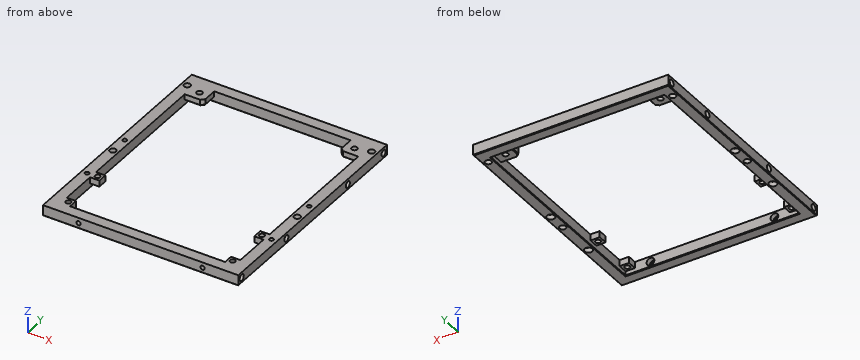
```python
from build123d import *

# Parameters (mm, degrees)
SKETCH1_W                       = 126
SKETCH1_H                       = 150
SKETCH1_W_2                     = 112
SKETCH1_H_2                     = 136
BOSS_EXTRUDE1_DEPTH             = 7
SKETCH2_R                       = 2.05
CUT_EXTRUDE1_DEPTH              = 6
SKETCH3_R                       = 1.35
CUT_EXTRUDE2_DEPTH              = 8
SKETCH4_R                       = 2.5
CUT_EXTRUDE3_DEPTH              = 3
SKETCH5_R                       = 1.35
CUT_EXTRUDE4_DEPTH              = 8
SKETCH6_R                       = 2.5
CUT_EXTRUDE5_DEPTH              = 3
SKETCH7_R                       = 2.05
CUT_EXTRUDE6_DEPTH              = 8
CUT_EXTRUDE7_DEPTH              = 0.2
SKETCH9_W                       = 2.7
SKETCH9_H                       = 2.7
CUT_EXTRUDE8_DEPTH              = 0.2
SKETCH10_W                      = 6
SKETCH10_H                      = 6
BOSS_EXTRUDE2_DEPTH             = 4
SKETCH11_R                      = 1.65
CUT_EXTRUDE9_DEPTH              = 5
CHAMFER1_SIZE                   = 0.4
CHAMFER2_SIZE                   = 0.4
SKIZZE2_W                       = 12
SKIZZE2_H                       = 11
SKIZZE2_R                       = 1.8
AUFSATZ_LINEAR_AUSTRAGEN1_DEPTH = 4
FASE1_SIZE                      = 2
FASE2_SIZE                      = 0.5


with BuildPart() as part:
    # Sketch1 → Boss-Extrude1 (new body)
    with BuildSketch(Plane.XY):
        Rectangle(SKETCH1_W, SKETCH1_H)
        Rectangle(SKETCH1_W_2, SKETCH1_H_2, mode=Mode.SUBTRACT)
    extrude(amount=BOSS_EXTRUDE1_DEPTH)

    # Sketch2 → Cut-Extrude1 (cut)
    with BuildSketch(Plane.ZY.offset(63)):
        with Locations((3.5, -71.5)):
            Circle(SKETCH2_R)
        with Locations((3.5, 71.5)):
            Circle(SKETCH2_R)
        with Locations((3.5, 35.5)):
            Circle(SKETCH2_R)
        with Locations((3.5, -26.5)):
            Circle(SKETCH2_R)
    cut_extrude1 = extrude(amount=-CUT_EXTRUDE1_DEPTH, mode=Mode.SUBTRACT)

    # Mirror1: Cut-Extrude1 across plane
    add(cut_extrude1.mirror(Plane(origin=(0, 0, 0), x_dir=(0, 0, 1), z_dir=(1, 0, 0))), mode=Mode.SUBTRACT)

    # Sketch3 → Cut-Extrude2 (cut, through all)
    with BuildSketch(Plane(origin=(0, -68, 0), x_dir=(1, 0, 0), z_dir=(0, 1, 0))):
        with Locations((40, -3.5)):
            Circle(SKETCH3_R)
        with Locations((-40, -3.5)):
            Circle(SKETCH3_R)
    extrude(amount=-CUT_EXTRUDE2_DEPTH, mode=Mode.SUBTRACT)

    # Sketch4 → Cut-Extrude3 (cut)
    with BuildSketch(Plane(origin=(0, -68, 0), x_dir=(1, 0, 0), z_dir=(0, 1, 0))):
        with Locations((40, -3.5)):
            Circle(SKETCH4_R)
        with Locations((-40, -3.5)):
            Circle(SKETCH4_R)
    extrude(amount=-CUT_EXTRUDE3_DEPTH, mode=Mode.SUBTRACT)

    # Sketch5 → Cut-Extrude4 (cut, through all)
    with BuildSketch(Plane(origin=(0, 0, 0), x_dir=(-1, 0, 0), z_dir=(0, 0, -1))):
        with Locations((-59.5, 2)):
            Circle(SKETCH5_R)
        with Locations((59.5, 2)):
            Circle(SKETCH5_R)
        with Locations((-59.5, -36)):
            Circle(SKETCH5_R)
        with Locations((59.5, -36)):
            Circle(SKETCH5_R)
    extrude(amount=-CUT_EXTRUDE4_DEPTH, mode=Mode.SUBTRACT)

    # Sketch6 → Cut-Extrude5 (cut)
    with BuildSketch(Plane(origin=(0, 0, 0), x_dir=(-1, 0, 0), z_dir=(0, 0, -1))):
        with Locations((-59.5, 2)):
            Circle(SKETCH6_R)
        with Locations((59.5, 2)):
            Circle(SKETCH6_R)
        with Locations((-59.5, -36)):
            Circle(SKETCH6_R)
        with Locations((59.5, -36)):
            Circle(SKETCH6_R)
    extrude(amount=-CUT_EXTRUDE5_DEPTH, mode=Mode.SUBTRACT)

    # Sketch7 → Cut-Extrude6 (cut, through all)
    with BuildSketch(Plane(origin=(0, 0, 0), x_dir=(-1, 0, 0), z_dir=(0, 0, -1))):
        with Locations((-59.5, 65)):
            Circle(SKETCH7_R)
        with Locations((-59.5, -10)):
            Circle(SKETCH7_R)
    cut_extrude6 = extrude(amount=-CUT_EXTRUDE6_DEPTH, mode=Mode.SUBTRACT)

    # Mirror2: Cut-Extrude6 across plane
    add(cut_extrude6.mirror(Plane(origin=(0, 0, 0), x_dir=(0, 0, 1), z_dir=(1, 0, 0))), mode=Mode.SUBTRACT)

    # Sketch8 → Cut-Extrude7 (cut)
    with BuildSketch(Plane(origin=(0, 0, 3), x_dir=(-1, 0, 0), z_dir=(0, 0, -1))):
        with BuildLine():
            Line((-60.85, -0.104162541), (-60.85, 4.104162541))
            ThreePointArc((-60.85, 4.104162541), (-59.5, 4.5), (-58.15, 4.104162541))
            Line((-58.15, 4.104162541), (-58.15, -0.104162541))
            ThreePointArc((-58.15, -0.104162541), (-59.5, -0.5), (-60.85, -0.104162541))
        make_face()
        with BuildLine():
            Line((-60.85, -38.104162541), (-60.85, -33.895837459))
            ThreePointArc((-60.85, -33.895837459), (-59.5, -33.5), (-58.15, -33.895837459))
            Line((-58.15, -33.895837459), (-58.15, -38.104162541))
            ThreePointArc((-58.15, -38.104162541), (-59.5, -38.5), (-60.85, -38.104162541))
        make_face()
    cut_extrude7 = extrude(amount=-CUT_EXTRUDE7_DEPTH, mode=Mode.SUBTRACT)

    # Sketch9 → Cut-Extrude8 (cut)
    with BuildSketch(Plane(origin=(0, 0, 3.2), x_dir=(-1, 0, 0), z_dir=(0, 0, -1))):
        with Locations((-59.5, 2)):
            Rectangle(SKETCH9_W, SKETCH9_H)
        with Locations((-59.5, -36)):
            Rectangle(SKETCH9_W, SKETCH9_H)
    cut_extrude8 = extrude(amount=-CUT_EXTRUDE8_DEPTH, mode=Mode.SUBTRACT)

    # Mirror3: Cut-Extrude7, Cut-Extrude8 across plane
    add(cut_extrude7.mirror(Plane(origin=(0, 0, 0), x_dir=(0, 0, 1), z_dir=(1, 0, 0))), mode=Mode.SUBTRACT)
    add(cut_extrude8.mirror(Plane(origin=(0, 0, 0), x_dir=(0, 0, 1), z_dir=(1, 0, 0))), mode=Mode.SUBTRACT)

    # Sketch10 → Boss-Extrude2 (add)
    with BuildSketch(Plane.XY.offset(7)):
        with Locations((53, -65)):
            Rectangle(SKETCH10_W, SKETCH10_H)
        with Locations((53, -35.5)):
            Rectangle(SKETCH10_W, SKETCH10_H)
    boss_extrude2 = extrude(amount=-BOSS_EXTRUDE2_DEPTH)

    # Sketch11 → Cut-Extrude9 (cut, through all)
    with BuildSketch(Plane(origin=(0, 0, 3), x_dir=(-1, 0, 0), z_dir=(0, 0, -1))):
        with Locations((-53, -35.5)):
            Circle(SKETCH11_R)
        with Locations((-53, -65)):
            Circle(SKETCH11_R)
    cut_extrude9 = extrude(amount=-CUT_EXTRUDE9_DEPTH, mode=Mode.SUBTRACT)

    # Mirror4: Boss-Extrude2, Cut-Extrude9 across plane
    add(boss_extrude2.mirror(Plane(origin=(0, 0, 0), x_dir=(0, 0, 1), z_dir=(1, 0, 0))))
    add(cut_extrude9.mirror(Plane(origin=(0, 0, 0), x_dir=(0, 0, 1), z_dir=(1, 0, 0))), mode=Mode.SUBTRACT)

    # Chamfer1
    chamfer1_edges = [part.edges().sort_by_distance(p)[0] for p in [
        (56, 0, 0),
        (0, 68, 0),
        (-56, 0, 0),
        (0, -68, 0),
    ]]
    chamfer(chamfer1_edges, length=CHAMFER1_SIZE)

    # Chamfer2
    chamfer2_edges = [part.edges().sort_by_distance(p)[0] for p in [
        (0, -75, 0),
        (-63, 0, 0),
        (0, 75, 0),
        (63, 0, 0),
    ]]
    chamfer(chamfer2_edges, length=CHAMFER2_SIZE)

    # Skizze2 → Aufsatz-Linear austragen1 (add)
    with BuildSketch(Plane.XY.offset(7)):
        with Locations((-50, 62.5)):
            Rectangle(SKIZZE2_W, SKIZZE2_H)
        with Locations((-50, 62.5)):
            Circle(SKIZZE2_R, mode=Mode.SUBTRACT)
        with Locations((50, 62.5)):
            Rectangle(SKIZZE2_W, SKIZZE2_H)
        with Locations((50, 62.5)):
            Circle(SKIZZE2_R, mode=Mode.SUBTRACT)
    extrude(amount=-AUFSATZ_LINEAR_AUSTRAGEN1_DEPTH)

    # Fase1
    fase1_edges = [part.edges().sort_by_distance(p)[0] for p in [
        (-44, 57, 5),
        (44, 57, 5),
    ]]
    chamfer(fase1_edges, length=FASE1_SIZE)

    # Fase2
    fase2_edges = [part.edges().sort_by_distance(p)[0] for p in [
        (-51, 57, 3),
        (44, 63.5, 3),
        (-44, 63.5, 3),
        (-45, 58, 3),
        (51, 57, 3),
        (45, 58, 3),
    ]]
    chamfer(fase2_edges, length=FASE2_SIZE)


solid = part.part
```
Check sheet for the modelled part. Datum: model origin and axes. Units: mm. Round coordinates to 2 decimals unless told otherwise and drop trailing zeros. Write each loop counter-clockwise with the first axis right and the second up, starting at its lowest first coordinate (ties: lowest second). Pieces come first, ordered by that corner, then holes. Notation, with made-up numbers: (77, 64) -> (133, 64) arc R27 cw to (133, 96) -> close; hole circle Ø10 at (58, 19). An arc over 180 degrees is marked (long way). Put each result on its own line as item: value.
(1) Material ranges on line 1 (X direction, y = 2, z = 0.95); line 2 (Y direction, x = -22.5, z = 6); line 3 (X direction, y = 60.5, z = 1), recorded low to high.
Values found:
line 1: x = -63 to -62, -57 to -56, 56 to 57, 62 to 63
line 2: y = -75 to -68, 68 to 75
line 3: x = -63 to -56, 56 to 63
(2) Go/stop test with flat-tipped pins: pin 1 Ø1.1 at (x, y) = (-60.5, -36.5) entering from -Z; pin 2 Ø2.5 at (x, y) = (-59.5, -10) entering from -Z. Record where each tip stops, or that it passes through.
Values found:
pin 1: stops at z = 3
pin 2: passes through
(3) Sectioned sample at B-B (x = -28). Enter the section's corners in (y, z).
Values found:
outline: (-75, 0.4) -> (-74.6, 0) -> (-68.4, 0) -> (-68, 0.4) -> (-68, 7) -> (-75, 7) -> close; (68, 0.4) -> (68.4, 0) -> (74.6, 0) -> (75, 0.4) -> (75, 7) -> (68, 7) -> close
(4) Sectioned sample at A-A (y = 19). Enter the section's corners in (x, z), plus the area to 3 significant figures.
Values found:
outline: (-63, 0.4) -> (-62.6, 0) -> (-56.4, 0) -> (-56, 0.4) -> (-56, 7) -> (-63, 7) -> close; (56, 0.4) -> (56.4, 0) -> (62.6, 0) -> (63, 0.4) -> (63, 7) -> (56, 7) -> close
area: 97.7 mm^2
(5) Sectioned sample at C-C (y = 35.5). Enter the section's corners in (x, z).
Values found:
outline: (-63, 0.4) -> (-62.6, 0) -> (-56.4, 0) -> (-56, 0.4) -> (-56, 7) -> (-63, 7) -> (-63, 5.55) -> (-57, 5.55) -> (-57, 1.45) -> (-63, 1.45) -> close; (56, 0.4) -> (56.4, 0) -> (62.6, 0) -> (63, 0.4) -> (63, 1.45) -> (57, 1.45) -> (57, 5.55) -> (63, 5.55) -> (63, 7) -> (56, 7) -> close
